The listing builds one solid part. Answer for the finished solid, in the listing's coordinates (mm). A direction names the side the tool comes from. Coordinates: 2 decimals unless noted, no trailing zeros. Loops run counter-clockwise (first coordinate to the right, second up) from the corner with the lowest first, then second, coordinate; pieces in that order, holes last. Notation, with made-up numbers: (-29, 19.5) - (-15, 19.5) arc R19 ccw to (-15, 46.5) - close; hole circle Ø9 at (49, 53.25). An arc over 180 degrees is marked (long way). Return JSON: item names as keys, results as strings. Group by question number.
1. Find the intervals of material crossed by line 1 along X through (y, z) = (12, 2.7); line 2 along X through (y, z) = (60.5, 2.6); line 3 along Y through (x, z) = (291, 1.8), in increasing order.
2. Section D-D (z = 1.1) is taken. State how many separate pieces and enclosed holes the cut face has, and give its area (3 significant figures).
3. Each of these flat-tipped pins is pushed along its axis until it touches: P1, Ø0.9, axis at y = 97.5, z = 1, coming from the +X side; P2, Ø4, axis at x = 105.5, y = 45.5, coming from the -Z side. Where does it stop, or does it pass through?
4. Section C-C (y = 100) is taken. Write down the section's boundary in (x, z), and give its area (3 significant figures).
5. Section A-A (x = 163.5) is taken. Write down the section's boundary in (y, z), and give its area (3 significant figures).
6. Section B-B (x = 50) is taken. Write down the section's boundary in (y, z), and give its area (3 significant figures).
7. Which of the six approach directions +Z, -Z, +X, -X, +Y, -Y give full straight-line access (tool end or side, diameter ignored) to faces 1 (the face through (213, 39, 0)), 2 (the face through (184.332, 100.335, 1.479))?
```python
from build123d import *

# Parameters (mm, degrees)
F0_R     = 2.25
F0_W     = 46.010702
F0_H     = 15.40207
F0_R_2   = 22.5
F0_R_3   = 1.75
F0_W_2   = 47.632419
F0_H_2   = 14.842443
F1_DEPTH = 3


with BuildPart() as f1:
    # F0 (on Top) → F1 (new body)
    with BuildSketch(Plane.XY):
        with BuildLine():
            Line((365, 135.2), (0, 75))
            Line((0, 75), (362.5, 75))
            ThreePointArc((362.5, 75), (363.232233, 76.767767), (365, 77.5))
            Line((365, 77.5), (365, 135.2))
        make_face()
        with BuildLine():
            Line((249.999995, 79.999998), (122.081561, 79.999998))
            ThreePointArc((122.081561, 79.999998), (117.098251, 84.591803), (121.267896, 89.933349))
            Line((121.267896, 89.933349), (249.18633, 111.031129))
            ThreePointArc((249.18633, 111.031129), (253.23509, 109.910148), (254.999995, 106.097778))
            Line((254.999995, 106.097778), (254.999995, 84.999998))
            ThreePointArc((254.999995, 84.999998), (253.535529, 81.464464), (249.999995, 79.999998))
        make_face(mode=Mode.SUBTRACT)
        with BuildLine():
            ThreePointArc((354.186335, 128.348938), (358.235095, 127.227957), (360, 123.415587))
            Line((360, 123.415587), (360, 84.999998))
            ThreePointArc((360, 84.999998), (358.535534, 81.464464), (355, 79.999998))
            Line((355, 79.999998), (270, 79.999998))
            ThreePointArc((270, 79.999998), (266.464466, 81.464464), (265, 84.999998))
            Line((265, 84.999998), (265, 109.396409))
            ThreePointArc((265, 109.396409), (266.18763, 112.631504), (269.186335, 114.32976))
            Line((269.186335, 114.32976), (354.186335, 128.348938))
        make_face(mode=Mode.SUBTRACT)
        with BuildLine():
            ThreePointArc((0, 5), (1.464466, 1.464466), (5, 0))
            Line((5, 0), (426.2, 0))
            ThreePointArc((426.2, 0), (429.735534, 1.464466), (431.2, 5))
            Line((431.2, 5), (431.2, 75))
            Line((431.2, 75), (367.5, 75))
            ThreePointArc((367.5, 75), (365, 72.5), (362.5, 75))
            Line((362.5, 75), (0, 75))
            Line((0, 75), (0, 5))
        make_face()
        with BuildLine():
            ThreePointArc((15, 10), (11.464466, 11.464466), (10, 15))
            Line((10, 15), (10, 60))
            ThreePointArc((10, 60), (11.464466, 63.535534), (15, 65))
            Line((15, 65), (177.248031, 65))
            Line((177.248031, 65), (177.248031, 65.195423))
            Line((177.248031, 65.195423), (221.969068, 65.195423))
            Line((221.969068, 65.195423), (221.969068, 65))
            Line((221.969068, 65), (276.665121, 65))
            Line((276.665121, 65), (291.45667, 65))
            Line((291.45667, 65), (346.2, 65))
            ThreePointArc((346.2, 65), (349.735534, 63.535534), (351.2, 60))
            Line((351.2, 60), (351.2, 56.482751))
            Line((351.2, 56.482751), (351.2, 16.981905))
            Line((351.2, 16.981905), (351.2, 15))
            ThreePointArc((351.2, 15), (349.735534, 11.464466), (346.2, 10))
            Line((346.2, 10), (291.45667, 10))
            Line((291.45667, 10), (277.253091, 10))
            Line((277.253091, 10), (123.603888, 10))
            Line((123.603888, 10), (123.603888, 9.868093))
            Line((123.603888, 9.868093), (74.839681, 9.868093))
            Line((74.839681, 9.868093), (74.839681, 10))
            Line((74.839681, 10), (15, 10))
        make_face(mode=Mode.SUBTRACT)
        with Locations((396.2, 15)):
            Circle(F0_R, mode=Mode.SUBTRACT)
        with Locations((396.2, 60)):
            Circle(F0_R, mode=Mode.SUBTRACT)
        with BuildLine():
            Line((10, 60), (10, 15))
            ThreePointArc((10, 15), (11.464466, 11.464466), (15, 10))
            Line((15, 10), (74.839681, 10))
            Line((74.839681, 10), (74.839681, 25.567258))
            Line((74.839681, 25.567258), (123.603888, 25.567258))
            Line((123.603888, 25.567258), (123.603888, 10))
            Line((123.603888, 10), (277.253091, 10))
            Line((277.253091, 10), (277.253091, 34.278966))
            Line((277.253091, 34.278966), (291.45667, 34.278966))
            Line((291.45667, 34.278966), (291.45667, 10))
            Line((291.45667, 10), (346.2, 10))
            ThreePointArc((346.2, 10), (349.735534, 11.464466), (351.2, 15))
            Line((351.2, 15), (351.2, 16.981905))
            Line((351.2, 16.981905), (313.055903, 16.981905))
            Line((313.055903, 16.981905), (313.055903, 56.482751))
            Line((313.055903, 56.482751), (351.2, 56.482751))
            Line((351.2, 56.482751), (351.2, 60))
            ThreePointArc((351.2, 60), (349.735534, 63.535534), (346.2, 65))
            Line((346.2, 65), (291.45667, 65))
            Line((291.45667, 65), (291.45667, 46.009973))
            Line((291.45667, 46.009973), (276.665121, 46.009973))
            Line((276.665121, 46.009973), (276.665121, 65))
            Line((276.665121, 65), (221.969068, 65))
            Line((221.969068, 65), (221.969068, 43.890707))
            Line((221.969068, 43.890707), (177.248031, 43.890707))
            Line((177.248031, 43.890707), (177.248031, 65))
            Line((177.248031, 65), (15, 65))
            ThreePointArc((15, 65), (11.464466, 63.535534), (10, 60))
        make_face()
        with Locations((200.134024, 17.866223)):
            Rectangle(F0_W, F0_H, mode=Mode.SUBTRACT)
        with Locations((50, 37.5)):
            Circle(F0_R_2, mode=Mode.SUBTRACT)
        with Locations((100, 37.5)):
            Circle(F0_R_3, mode=Mode.SUBTRACT)
        with Locations((99.295299, 57.364914)):
            Rectangle(F0_W_2, F0_H_2, mode=Mode.SUBTRACT)
        with Locations((150, 37.5)):
            Circle(F0_R_2, mode=Mode.SUBTRACT)
        with Locations((200, 37.5)):
            Circle(F0_R_3, mode=Mode.SUBTRACT)
        with Locations((250, 37.5)):
            Circle(F0_R_2, mode=Mode.SUBTRACT)
        with Locations((300, 37.5)):
            Circle(F0_R_3, mode=Mode.SUBTRACT)
    extrude(amount=F1_DEPTH)


solid = f1.part
```
The answers:
{
 "1": {"line 1": "x = 0 to 74.84, 123.6 to 177.13, 223.14 to 277.25, 291.46 to 431.2", "line 2": "x = 0 to 75.48, 123.11 to 177.25, 221.97 to 276.67, 291.46 to 394.01, 398.39 to 431.2", "line 3": "y = 0 to 10, 34.28 to 46.01, 65 to 80, 117.93 to 123"},
 "2": {"separate pieces": "1", "enclosed holes": "17", "area": "26,500 mm2"},
 "3": {"P1": "stops at x = 365", "P2": "stops at z = 0"},
 "4": {"outline": "(151.58, 0) - (182.3, 0) - (182.3, 3) - (151.58, 3) - close; (255, 0) - (265, 0) - (265, 3) - (255, 3) - close; (360, 0) - (365, 0) - (365, 3) - (360, 3) - close", "area": "137 mm2"},
 "5": {"outline": "(0, 0) - (19.5, 0) - (19.5, 3) - (0, 3) - close; (55.5, 0) - (80, 0) - (80, 3) - (55.5, 3) - close; (96.9, 0) - (101.97, 0) - (101.97, 3) - (96.9, 3) - close", "area": "147 mm2"},
 "6": {"outline": "(0, 0) - (15, 0) - (15, 3) - (0, 3) - close; (60, 0) - (83.25, 0) - (83.25, 3) - (60, 3) - close", "area": "115 mm2"},
 "7": {"face 1": "-Z, +X, -X, +Y, -Y", "face 2": "+Z, -Z"}
}
